Part model, mm, in its own coordinate system. Face numbers are marked on the shaded views. A direction names the side the tool comes from. Round coordinates to 2 decimals unless told otherwise and drop trailing zeros. Loops run counter-clockwise (first coordinate to the right, second up) from the corner with the lowest first, then second, coordinate; pieces in that order, holes last. Notation, with made-up numbers: M -38,-31.5 L -2,-31.5 A28 ccw -2,-3.5 Z; hole C 62.25,31 d1. An arc over 180 degrees is marked long. Put each result on its own line as item: value. Start each with the question number.
1) Slice it at D-D on y = 225.5. Give the cut face in (x, z).
2) Probe line 1 along Z through (x, y) = (0, 250.95); line 2 along X through (y, z) = (250.9, 15); line 3 along Y through (x, z) = (-5, 0). List the from-to ranges inside material, lowest first.
3) Slice it at C-C on y = 125. Give the cut face in (x, z), then the cut area to 3 significant figures.
4) Slice it at A-A on z = 0. Give the cut face in (x, y), then the cut area to 3 significant figures.
5) Pull direction Y, two halves, no side cores. Call the marked faces 1, 2 and 3: +Y half, -Y half, draft (parallel to the pull), parting line (faces both ways), or undercut.
6) Slice it at B-B on x = -6.75. Give the cut face in (y, z), then the cut area to 3 significant figures.
7) Drop flat-ended pins along their axis: pin 1 Ø3 at (x, y) = (-6, 76) entering from -Z; pin 2 Ø1.5 at (x, y) = (3, 45) entering from +Z; pin 3 Ø2.5 at (x, y) = (4.5, 3.5) entering from +Z. Give the stop position or say it passes through.
8) Which spindle directions (+Z, -Z, +X, -X, +Y, -Y) get a long thin tool onto all of the face, cutting with end or side? Do the marked faces 4, 5 and 6. Say none if no direction does.
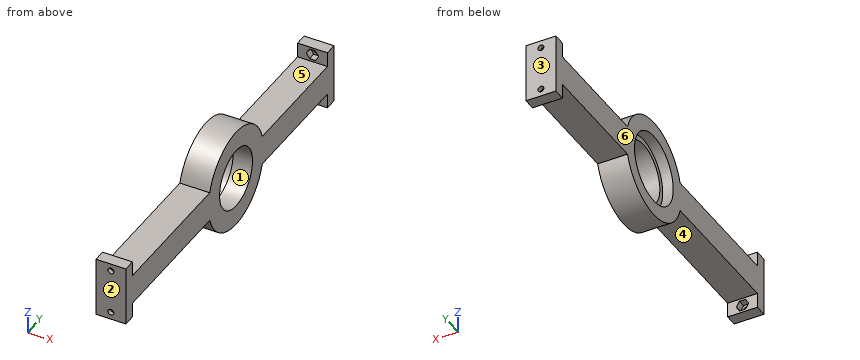
Autodesk Inventor part; units mm, degrees
ref_plane "YZ Plane" through (0, 0, 0) normal (1, 0, 0) x (0, 1, 0)
ref_plane "XZ Plane" through (0, 0, 0) normal (0, 1, 0) x (-1, 0, 0)
ref_plane "XY Plane" through (0, 0, 0) normal (0, 0, 1) x (1, 0, 0)
sketch "Sketch4" plane through (0, 0, 0) normal (0, 1, 0) x (-1, 0, 0)
  line L0 (-10, 20) -> (10, 20)
  line L1 (10, 20) -> (10, -20)
  line L2 (10, -20) -> (-10, -20)
  line L3 (-10, -20) -> (-10, 20)
  line L4 (-10, 20) -> (10, -20) construction
  line L5 (10, 20) -> (-10, -20) construction
  point P0 (0, 0)
  dimension "d8" = 20
  dimension "d9" = 40
extrude "Extrusion2" add sketch "Sketch4" along normal blind 3
sketch "Sketch5" plane through (0, 3, 0) normal (0, 1, 0) x (1, 0, 0)
  line L0 (10, -10) -> (-10, -10)
  line L1 (-10, -10) -> (-10, 10)
  line L2 (-10, 10) -> (10, 10)
  line L3 (10, 10) -> (10, -10)
  line L4 (10, -10) -> (-10, 10) construction
  line L5 (-10, -10) -> (10, 10) construction
  point P0 (0, 0)
  dimension "d12" = 20
  dimension "d13" = 20
extrude "Extrusion3" add sketch "Sketch5" along normal blind 100
sketch "Sketch7" plane through (0, 3, 0) normal (0, 1, 0) x (1, 0, 0)
  circle A0 centre (0, 15) radius 2
  circle A1 centre (0, -15) radius 2
  point P0 (0, 0)
  dimension "d20" = 4
  dimension "d21" = 4
extrude "Extrusion5" cut sketch "Sketch7" against normal blind 10
sketch "Sketch8" plane through (0, 3, 0) normal (0, 1, 0) x (1, 0, 0)
  circle A0 centre (0, 15) radius 2
  circle A1 centre (0, 15) radius 3.55
  circle A2 centre (0, -15) radius 2
  circle A3 centre (0, -15) radius 3.55
  line L0 (2.0496, -11.45) -> (4.0992, -15)
  line L1 (4.0992, -15) -> (2.0496, -18.55)
  line L2 (2.0496, -18.55) -> (-2.0496, -18.55)
  line L3 (-2.0496, -18.55) -> (-4.0992, -15)
  line L4 (-4.0992, -15) -> (-2.0496, -11.45)
  line L5 (-2.0496, -11.45) -> (2.0496, -11.45)
  line L6 (2.0496, 18.55) -> (4.0992, 15)
  line L7 (4.0992, 15) -> (2.0496, 11.45)
  line L8 (2.0496, 11.45) -> (-2.0496, 11.45)
  line L9 (-2.0496, 11.45) -> (-4.0992, 15)
  line L10 (-4.0992, 15) -> (-2.0496, 18.55)
  line L11 (-2.0496, 18.55) -> (2.0496, 18.55)
  point P0 (0, 0)
  point P1 (0, -11.45)
  point P2 (0, 18.55)
  dimension "d24" = 7.1
  dimension "d25" = 7.1
extrude "Extrusion6" cut sketch "Sketch8" against normal blind 3 contours A0 | A1 | A1 L6 L7 | A1 L11 L6 | L7 L8 A1 | A1 L10 L11 | L8 L9 A1 | A1 L9 L10 | A2 | A3 | A3 L0 L1 | A3 L5 L0 | L1 L2 A3 | A3 L4 L5 | L2 L3 A3 | A3 L3 L4
sketch "Sketch9" plane through (0, 0, 0) normal (0, -1, 0) x (1, 0, 0)
  line L0 (2.0496, 11.45) -> (4.0992, 15)
  circle A0 centre (0, 15) radius 4.0992
  circle A1 centre (0, -15) radius 4.0992
  point P0 (0, 0)
  point P1 (4.0992, -15)
sketch "Sketch11" plane through (-10, 0, -20) normal (-1, 0, 0) x (0, 0, 1)
  line L0 (10, 0) -> (30, 0)
  line L1 (30, 0) -> (30, 250)
  line L2 (30, 250) -> (10, 250)
  line L3 (10, 250) -> (10, 0)
  arc A0 (29.9121, 100) -> (10.0879, 100) centre (20, 132) ccw
  line L4 (10, 250) -> (30, 250)
  line L5 (30, 250) -> (30, 163.9726)
  line L6 (30, 163.9726) -> (10, 163.9726)
  line L7 (10, 163.9726) -> (10, 250)
  point P0 (20, 0)
  point P1 (10, 163.9726)
  dimension "d29" = 250
extrude "Extrusion7" add sketch "Sketch11" against normal blind 20 contours L3 L2 L1 A0
sketch "Sketch14" plane through (-10, 250, 10) normal (0, 1, 0) x (1, 0, 0)
  line L0 (0, 0) -> (0, -10)
  line L1 (20, -10) -> (20, 30)
  line L2 (0, -10) -> (20, -10)
  line L3 (20, -10) -> (20, 30)
  line L4 (20, 30) -> (0, 30)
  line L5 (0, 30) -> (0, -10)
  point P0 (10, 10)
extrude "Extrusion8" add sketch "Sketch14" along normal blind 3
sketch "Sketch15" plane through (-10, 253, 10) normal (0, 1, 0) x (1, 0, 0)
  circle A0 centre (10, 25) radius 3.5
  circle A1 centre (10, -5) radius 3.5
  line L0 (12.0207, 28.5) -> (14.0415, 25)
  line L1 (14.0415, 25) -> (12.0207, 21.5)
  line L2 (12.0207, 21.5) -> (7.9793, 21.5)
  line L3 (7.9793, 21.5) -> (5.9585, 25)
  line L4 (5.9585, 25) -> (7.9793, 28.5)
  line L5 (7.9793, 28.5) -> (12.0207, 28.5)
  line L6 (12.0207, -1.5) -> (14.0415, -5)
  line L7 (14.0415, -5) -> (12.0207, -8.5)
  line L8 (12.0207, -8.5) -> (7.9793, -8.5)
  line L9 (7.9793, -8.5) -> (5.9585, -5)
  line L10 (5.9585, -5) -> (7.9793, -1.5)
  line L11 (7.9793, -1.5) -> (12.0207, -1.5)
  point P0 (10, 10)
  point P1 (10, 28.5)
  point P2 (10, -1.5)
  dimension "d34" = 7
  dimension "d35" = 7
extrude "Extrusion9" cut sketch "Sketch15" against normal blind 3
sketch "Sketch16" plane through (-10, 253, 10) normal (0, 1, 0) x (1, 0, 0)
  line L0 (12.0207, 21.5) -> (14.0415, 25)
  circle A0 centre (10, 25) radius 4.0415
  line L1 (7.9793, -1.5) -> (12.0207, -1.5)
  circle A1 centre (10, -5) radius 4.0415
  point P0 (10, 10)
sketch "Sketch17" plane through (10, 0, 20) normal (1, 0, 0) x (0, 0, -1)
  circle A0 centre (20, 133.9) radius 23.5
  circle A1 centre (20, 133.9) radius 33.5
  point P0 (20, 0)
  dimension "d38" = 47
  dimension "d39" = 67
extrude "Extrusion10" add sketch "Sketch17" against normal blind 20
sketch "Sketch18" plane through (10, 0, 20) normal (1, 0, 0) x (0, 0, -1)
  point P0 (20, 0)
sketch "Sketch19" plane through (10, 0, 20) normal (1, 0, 0) x (0, 0, -1)
  circle A0 centre (20, 133.9) radius 23.5
  circle A1 centre (20, 133.9) radius 20
  point P0 (20, 0)
  dimension "d42" = 40
extrude "Extrusion11" add sketch "Sketch19" against normal blind 13
thicken "Thicken1" operation add thickness 5 both sides no extend neighbours yes toward (0, 1, 0) faces at (8.0331, 3, 15) (8.0331, 3, -15)
sketch "Sketch20" plane through (0, 0, 0) normal (0, -1, 0) x (1, 0, 0)
  line L0 (-10, 20) -> (10, 20)
  line L1 (10, -20) -> (-10, -20)
  line L2 (-10, 20) -> (10, 20)
  line L3 (10, 20) -> (10, -20)
  line L4 (10, -20) -> (-10, -20)
  line L5 (-10, -20) -> (-10, 20)
  point P0 (0, 0)
extrude "Extrusion12" add sketch "Sketch20" against normal blind 3
sketch "Sketch21" plane through (0, 3, 0) normal (0, 1, 0) x (1, 0, 0)
  circle A0 centre (0, -15) radius 2
  circle A1 centre (0, 15) radius 2
  point P0 (0, 0)
  dimension "d49" = 4
  dimension "d50" = 4
extrude "Extrusion13" cut sketch "Sketch21" against normal blind 3
thicken "Thicken2" operation add thickness 5 both sides no extend neighbours yes toward (0, -1, 0) faces at (8.0138, 250, -15) (8.0138, 250, 15)
sketch "Sketch22" plane through (-10, 253, 10) normal (0, 1, 0) x (1, 0, 0)
  line L0 (0, -10) -> (20, -10)
  line L1 (20, 30) -> (0, 30)
  line L2 (0, -10) -> (20, -10)
  line L3 (20, -10) -> (20, 30)
  line L4 (20, 30) -> (0, 30)
  line L5 (0, 30) -> (0, -10)
  point P0 (10, 10)
extrude "Extrusion14" add sketch "Sketch22" against normal blind 3
sketch "Sketch23" plane through (-10, 253, 10) normal (0, 1, 0) x (1, 0, 0)
  circle A0 centre (10, -5) radius 2
  circle A1 centre (10, -5) radius 2
  circle A2 centre (10, 25) radius 2
  circle A3 centre (10, 25) radius 2
  point P0 (10, 10)
  dimension "d57" = 4
  dimension "d58" = 4
extrude "Extrusion15" cut sketch "Sketch23" against normal blind 3
properties part number "pylon"
Recorded:
1. outline: M -10,-10 L 10,-10 L 10,10 L -10,10 Z
2. line 1: z = -20 to -17, -13 to 13, 17 to 20
2. line 2: x = -10 to -2, 2 to 10
2. line 3: y = 0 to 110.4, 157.4 to 253
3. outline: M -10,-32.3 L 10,-32.3 L 10,-17.91 L -3,-17.91 L -3,-21.75 L -10,-21.75 Z; M -10,21.75 L -3,21.75 L -3,17.91 L 10,17.91 L 10,32.3 L -10,32.3 Z
3. area: 522 mm2
4. outline: M -10,0 L 10,0 L 10,113.9 L -3,113.9 L -3,110.4 L -10,110.4 Z; M -10,157.4 L -3,157.4 L -3,153.9 L 10,153.9 L 10,253 L -10,253 Z
4. area: 4,210 mm2
5. face 1: undercut
5. face 2: -Y half
5. face 3: +Y half
6. outline: M 0,-20 L 8,-20 L 8,-10 L 101.93,-10 A33.5 ccw 165.87,-10 L 245,-10 L 245,-20 L 253,-20 L 253,20 L 245,20 L 245,10 L 165.87,10 A33.5 ccw 101.93,10 L 8,10 L 8,20 L 0,20 Z; hole C 133.9,0 d47
6. area: 5,850 mm2
7. pin 1: stops at z = -10
7. pin 2: stops at z = 10
7. pin 3: stops at z = 20
8. face 4: -Z, +X, -X
8. face 5: +Z, +X, -X
8. face 6: +Z, -Z, -X, +Y, -Y
